The model under review builds one solid part; all positions refer to its coordinate system, in mm. Face numbers are marked on the shaded views. A direction names the side the tool comes from. Round coordinates to 2 decimals unless told otherwise and drop trailing zeros. Write each loop counter-clockwise with the first axis right and the second up, starting at its lowest first coordinate (ties: lowest second). Pieces come first, ordered by that corner, then holes. Notation, with made-up numbers: (28.5, 86) -> (37.5, 86) arc R35 cw to (37.5, 118) -> close; hole circle Ø4 at (12.25, 79.25). An arc over 180 degrees is marked (long way). Answer as a JSON object with one key per item and string values. Group by question number.
1) Insertion check: pin 1 Ø4 at (x, y) = (-1.5, 5.5) entering from -Z; pin 2 Ø3 at (y, z) = (4, 5.5) entering from -X; pin 3 Ø6.5 at (x, z) = (0, 0) entering from +Y; pin 4 Ø2 at (y, z) = (7.5, 6.5) entering from -X. Each pin has a flat end and moves straight along its axis. Give the tip position at first contact, or say it passes through.
2) We need section D-D, the plane z = 6.5. Write out the cut boundary in (x, y).
3) We need section A-A, the plane y = 4. Write out the cut boundary in (x, z), then the cut area to 3 significant figures.
4) Mouldability with a two-part tool opening along Y and no side actions: class the marked faces 4, 5 and 6 as pulls with the +Y half, pulls with the -Y half, needs draft (parallel to the pull), parting line crosses it, or undercut.
5) To check wall thickness, follow probe 1 along Y at (x, z) = (4, 9); probe 2 along Z at (x, y) = (-0.25, 2). State the ranges of each line that lie inside material, in increasing order. Write a range as [from, to].
6) We need section C-C, the plane z = -9.75. Write out the cut boundary in (x, y).
7) We need section B-B, the plane x = 9.75. Write out the cut boundary in (y, z), then the cut area to 3 significant figures.
8) Machinability: for the marked faces 1, 2 and 3, which of the approach directions +Z, -Z, +X, -X, +Y, -Y give a long, thin tool a straight path to every point of the face, cutting with its end or side? Answer none if there is none.
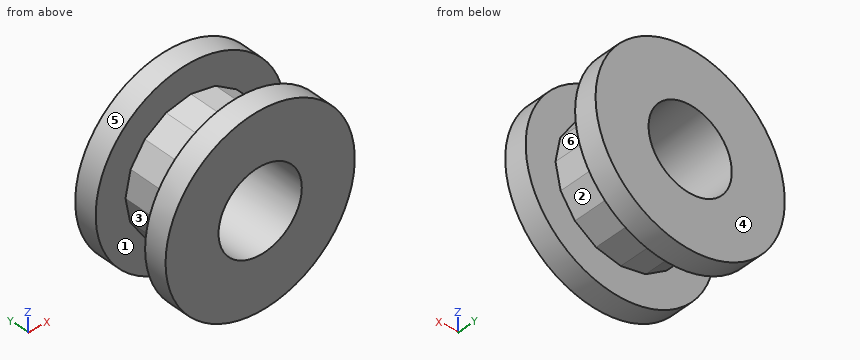
Autodesk Inventor part; units mm, degrees
ref_plane "YZ Plane" through (0, 0, 0) normal (1, 0, 0) x (0, 1, 0)
ref_plane "XZ Plane" through (0, 0, 0) normal (0, 1, 0) x (-1, 0, 0)
ref_plane "XY Plane" through (0, 0, 0) normal (0, 0, 1) x (1, 0, 0)
sketch "Szkic1" plane through (0, 0, 0) normal (0, 1, 0) x (-1, 0, 0)
  circle A0 centre (0, 0) radius 12.5
  dimension "d0" = 25
extrude "Wyciągnięcie proste1" add sketch "Szkic1" along normal blind 3
sketch "Szkic7" plane through (0, 3, 0) normal (0, 1, 0) x (1, 0, 0)
  line L0 (6, 6.109) -> (7.8811, 3.3479)
  line L1 (7.8811, 3.3479) -> (8.5624, 0.0771)
  line L2 (8.5624, 0.0771) -> (7.9401, -3.2055)
  line L3 (7.9401, -3.2055) -> (6.109, -6)
  line L4 (6.109, -6) -> (3.3479, -7.8811)
  line L5 (3.3479, -7.8811) -> (0.0771, -8.5624)
  line L6 (0.0771, -8.5624) -> (-3.2055, -7.9401)
  line L7 (-3.2055, -7.9401) -> (-6, -6.109)
  line L8 (-6, -6.109) -> (-7.8811, -3.3479)
  line L9 (-7.8811, -3.3479) -> (-8.5624, -0.0771)
  line L10 (-8.5624, -0.0771) -> (-7.9401, 3.2055)
  line L11 (-7.9401, 3.2055) -> (-6.109, 6)
  line L12 (-6.109, 6) -> (-3.3479, 7.8811)
  line L13 (-3.3479, 7.8811) -> (-0.0771, 8.5624)
  line L14 (-0.0771, 8.5624) -> (3.2055, 7.9401)
  line L15 (3.2055, 7.9401) -> (6, 6.109)
  point P0 (0, 0)
  point P1 (0, 0)
extrude "Wyciągnięcie proste6" add sketch "Szkic7" along normal blind 7.25
sketch "Szkic8" plane through (0, 10.25, 0) normal (0, 1, 0) x (1, 0, 0)
  circle A0 centre (0, 0) radius 12.5
extrude "Wyciągnięcie proste7" add sketch "Szkic8" along normal blind 3
sketch "Szkic9" plane through (0, 13.25, 0) normal (0, 1, 0) x (1, 0, 0)
  circle A0 centre (0, 0) radius 5.5016
extrude "Wyciągnięcie proste8" cut sketch "Szkic9" against normal blind 30
properties part number "spool_short"
Here are the results:
{
 "1": {"pin 1": "stops at z = -8.56", "pin 2": "stops at x = -11.71", "pin 3": "passes through", "pin 4": "stops at x = -6.41"},
 "2": {"outline": "(-10.68, 0) -> (10.68, 0) -> (10.68, 3) -> (5.38, 3) -> (5.38, 10.25) -> (10.68, 10.25) -> (10.68, 13.25) -> (-10.68, 13.25) -> (-10.68, 10.25) -> (-5.4, 10.25) -> (-5.4, 3) -> (-10.68, 3) -> close"},
 "3": {"outline": "(-8.56, 0.08) -> (-7.94, -3.21) -> (-6.11, -6) -> (-3.35, -7.88) -> (-0.08, -8.56) -> (3.21, -7.94) -> (6, -6.11) -> (7.88, -3.35) -> (8.56, -0.08) -> (7.94, 3.21) -> (6.11, 6) -> (3.35, 7.88) -> (0.08, 8.56) -> (-3.21, 7.94) -> (-6, 6.11) -> (-7.88, 3.35) -> close; hole circle Ø11 at (0, 0)", "area": "129 mm^2"},
 "4": {"face 4": "pulls with the +Y half", "face 5": "needs draft", "face 6": "undercut"},
 "5": {"probe 1": "y = [0, 3], [10.25, 13.25]", "probe 2": "z = [-12.5, -5.5], [5.5, 12.5]"},
 "6": {"outline": "(-7.82, 0) -> (7.82, 0) -> (7.82, 3) -> (-7.82, 3) -> close; (-7.82, 10.25) -> (7.82, 10.25) -> (7.82, 13.25) -> (-7.82, 13.25) -> close"},
 "7": {"outline": "(0, -7.82) -> (3, -7.82) -> (3, 7.82) -> (0, 7.82) -> close; (10.25, -7.82) -> (13.25, -7.82) -> (13.25, 7.82) -> (10.25, 7.82) -> close", "area": "93.9 mm^2"},
 "8": {"face 1": "none", "face 2": "-Z, +X", "face 3": "-Z, -X"}
}
